Input: part model. Units: mm. Frame: model coordinates. A direction names the side the tool comes from. Round coordinates to 2 decimals unless told otherwise and drop trailing zeros. Loops run counter-clockwise (first coordinate to the right, second up) from the corner with the lowest first, then second, coordinate; pieces in that order, holes last. Notation, with made-up numbers: (-20.5, 58.25) -> (31.5, 58.25) arc R32 cw to (31.5, 85.25) -> close; hole circle Ø9 at (25, -33). An arc over 180 degrees is marked (long way). Answer as a JSON object with one key per item and string values.
```python
from build123d import *

# Parameters (mm, degrees)
BOSS_EXTRUDE1_DEPTH = 20
SKETCH3_R           = 5
BOSS_EXTRUDE2_DEPTH = 20
CUT_EXTRUDE1_DEPTH  = 10


with BuildPart() as part:
    # Sketch2 → Boss-Extrude1 (new body)
    with BuildSketch(Plane(origin=(0, 0, 0), x_dir=(1, 0, 0), z_dir=(0, 1, 0))):
        Polygon((-0.85, 2.3), (0.85, 2.3), (0.85, 0.85), (2.3, 0.85), (2.3, -0.85), (0.85, -0.85), (0.85, -2.3), (-0.85, -2.3), (-0.85, -0.85), (-2.3, -0.85), (-2.3, 0.85), (-0.85, 0.85), align=None)
    extrude(amount=BOSS_EXTRUDE1_DEPTH)

    # Sketch3 → Boss-Extrude2 (add)
    with BuildSketch(Plane(origin=(0, 20, 0), x_dir=(1, 0, 0), z_dir=(0, 1, 0))):
        with Locations(Location((0, 0, 0), (0, 0, 270))):
            Circle(SKETCH3_R)
    extrude(amount=BOSS_EXTRUDE2_DEPTH)

    # Sketch4 → Cut-Extrude1 (cut)
    with BuildSketch(Plane(origin=(0, 40, 0), x_dir=(1, 0, 0), z_dir=(0, 1, 0))):
        with BuildLine():
            Line((-1.125, -0.992156742), (1.125, -0.992156742))
            ThreePointArc((1.125, -0.992156742), (0, 1.5), (-1.125, -0.992156742))
        make_face()
    extrude(amount=-CUT_EXTRUDE1_DEPTH, mode=Mode.SUBTRACT)


solid = part.part
```
1) Draft query along X for faces 4 (the face through (-0.85, 10, -2)), 5 (the face through (-4.88, 29.86, -1.08)), 6 (the face through (-1, 20, 1)), 7 (the face through (0, 35.1, -1.5)). Return one class per face: +X half, -X half, draft (parallel to the pull), parting line (faces both ways), or undercut.
Output:
{"face 4": "-X half", "face 5": "parting line", "face 6": "draft", "face 7": "undercut"}
2) Ray query, probe 1 along X at (y, z) = (37.75, 0); probe 2 along Y at (x, z) = (-2.5, -0.5); probe 3 along Z at (x, y) = (1.5, 14.5). Return the intervals inside material, ascending.
Output:
{"probe 1": "x = -5 to -1.5, 1.5 to 5", "probe 2": "y = 20 to 40", "probe 3": "z = -0.85 to 0.85"}
3) Reachability of faces 1 (the face through (-2.3, 10, 0)), 2 (the face through (2.3, 10, 0)), 3 (the face through (2, 10, 0.85)) from +Z, -Z, +X, -X, +Y, -Y: full face, straight path, thin tool, end or side. Return the list, or none.
Output:
{"face 1": "+Z, -Z, -X, -Y", "face 2": "+Z, -Z, +X, -Y", "face 3": "+Z, +X, -Y"}
4) Section D-D, the plane x = -4. Output: boundary loops of the cut face in (y, z).
Output:
{"outline": "(20, -3) -> (40, -3) -> (40, 3) -> (20, 3) -> close"}
5) Section A-A, the plane z = 0. Output: boundary loops of the cut face in (x, y).
Output:
{"outline": "(-5, 20) -> (-2.3, 20) -> (-2.3, 0) -> (2.3, 0) -> (2.3, 20) -> (5, 20) -> (5, 40) -> (1.5, 40) -> (1.5, 30) -> (-1.5, 30) -> (-1.5, 40) -> (-5, 40) -> close"}
6) Section B-B, the plane x = 0. Output: boundary loops of the cut face in (y, z).
Output:
{"outline": "(0, -2.3) -> (20, -2.3) -> (20, -5) -> (40, -5) -> (40, -1.5) -> (30, -1.5) -> (30, 0.99) -> (40, 0.99) -> (40, 5) -> (20, 5) -> (20, 2.3) -> (0, 2.3) -> close"}
7) Contact query for flat-ended pins moving along their axis: P1, Ø1.2, axis at x = 1.5, y = 10, coming from the -Z side; P2, Ø1.4, axis at x = 0, y = 8.5, coming from the -Z side; P3, Ø5, axis at x = -0.5, z = 0, coming from the -Y side; P4, Ø1.2, axis at y = 8.5, z = -1.5, coming from the +X side. Output: stop coordinate, or through.
Output:
{"P1": "stops at z = -0.85", "P2": "stops at z = -2.3", "P3": "stops at y = 0", "P4": "stops at x = 0.85"}
8) Section C-C, the plane y = 26. Output: boundary loops of the cut face in (x, z).
Output:
{"outline": "circle Ø10 at (0, 0)"}
